Autodesk Inventor part; units mm, degrees
ref_plane "YZ Plane" through (0, 0, 0) normal (1, 0, 0) x (0, 1, 0)
ref_plane "XZ Plane" through (0, 0, 0) normal (0, 1, 0) x (-1, 0, 0)
sketch "Sketch1" plane through (0, 0, 0) normal (0, 1, 0) x (-1, 0, 0)
  line L0 (25.4, 127) -> (-25.4, 127)
  line L1 (-25.4, 127) -> (-25.4, -127)
  line L2 (-25.4, -127) -> (25.4, -127)
  line L3 (25.4, -127) -> (25.4, 127)
  line L4 (25.4, 127) -> (-25.4, -127) construction
  line L5 (-25.4, 127) -> (25.4, -127) construction
  point P0 (0, 0)
  dimension "d0" = 50.8
  dimension "d1" = 254
extrude "Extrusion1" add sketch "Sketch1" along normal blind 25.4
sketch "Sketch2" plane through (0, 0, 0) normal (0, -1, 0) x (1, 0, 0)
  line L0 (-25.4, 127) -> (-25.4, 114.3)
  line L1 (-25.4, 114.3) -> (25.4, 114.3)
  line L2 (25.4, 114.3) -> (25.4, 127)
  line L3 (25.4, 127) -> (-25.4, 127)
  line L4 (-25.4, 127) -> (25.4, 114.3) construction
  line L5 (-25.4, 114.3) -> (25.4, 127) construction
  line L6 (-25.4, 127) -> (25.4, 127)
  point P0 (0, 0)
  point P1 (0, 120.65)
  dimension "d4" = 12.7
  dimension "d5" = 25.4
  dimension "d6" = 0
extrude "Extrusion2" add sketch "Sketch2" along normal blind 6.35
mirror "Mirror1" about plane through (0, 0, 0) normal (0, 0, 1) of "Extrusion2"
sketch "Sketch3" plane through (0, 25.4, 0) normal (0, 1, 0) x (1, 0, 0)
  circle A0 centre (0, -88.9) radius 4.7625
  line L0 (-25.4, -127) -> (25.4, -127)
  point P0 (0, 0)
  dimension "d9" = 9.525
  dimension "d10" = 38.1
extrude "Extrusion3" cut sketch "Sketch3" against normal through all
mirror "Mirror2" about plane through (0, 0, 0) normal (0, 0, 1) of "Extrusion3"
sketch "Sketch4" plane through (0, 25.4, 0) normal (0, 1, 0) x (1, 0, 0)
  line L0 (-15.875, -76.2) -> (15.875, -76.2)
  line L1 (15.875, -76.2) -> (15.875, 76.2)
  line L2 (15.875, 76.2) -> (-15.875, 76.2)
  line L3 (-15.875, 76.2) -> (-15.875, -76.2)
  line L4 (-15.875, -76.2) -> (15.875, 76.2) construction
  line L5 (15.875, -76.2) -> (-15.875, 76.2) construction
  line L6 (-25.4, 127) -> (-25.4, -127)
  line L7 (-25.4, -127) -> (25.4, -127)
  point P0 (0, 0)
  dimension "d13" = 9.525
  dimension "d14" = 50.8
extrude "Extrusion4" cut sketch "Sketch4" against normal through all
properties part number "BandSawJigTop" material "LCP Plastic"
The model under review builds one solid part; all positions refer to its coordinate system, in mm. A direction names the side the tool comes from. Round coordinates to 2 decimals unless told otherwise and drop trailing zeros. Write each loop counter-clockwise with the first axis right and the second up, starting at its lowest first coordinate (ties: lowest second). Pieces come first, ordered by that corner, then holes. Notation, with made-up numbers: (56.5, -2.5) - (105.5, -2.5) arc R25 ccw to (105.5, 15.5) - close; hole circle Ø6 at (-32, 79.5). An arc over 180 degrees is marked (long way). One line per item, written item: value. Start each with the question number.
1. The part is to be moulded in two halves that separate along X. For faces 1 (the face through (0, 13, 76.2)), 2 (the face through (0, -3, 114.3)), 3 (the face through (15.875, 13, 1)), 4 (the face through (-25.4, 13, 2)), say which applies: released by +X, released by -X, zero draft, split by the parting line, or undercut.
2. Machinability: for faces 5 (the face through (-17, 25.4, 2)), 6 (the face through (0, 13, -76.2)), 7 (the face through (0, -3, -114.3)), which of the approach directions +Z, -Z, +X, -X, +Y, -Y give a long, thin tool a straight path to every point of the face, cutting with its end or side? Answer none if there is none.
3. Clearance check with a flat-ended pin moving along its axis: P1, Ø15, axis at x = 10.5, z = 26.5, coming from the -Y side. State where the tip first meets the part, or that it passes through.
4. Consider section D-D on y = -3. Write out the cut boundary in (x, z), and give its area (3 significant figures).
5. To check wall thickness, follow L1, parallel to Z at x = 0, y = 17.5; L2, parallel to X at y = 13, z = 35.5 (3 decimals); L3, parallel to Z at x = 11.5, y = -3. State the ranges of each line that lie inside material, in increasing order. Write a range as from..to.
6. Consider section C-C on y = 21. Write out the cut boundary in (x, z) (1 decimal).
7. Consider section B-B on z = -25. Write out the cut boundary in (x, y) (3 decimals).
8. Consider section A-A on x = 8. Write out the cut boundary in (y, z).
Checks:
1. face 1: undercut
1. face 2: zero draft
1. face 3: undercut
1. face 4: released by -X
2. face 5: +Z, -Z, +X, -X, +Y
2. face 6: +Y, -Y
2. face 7: +X, -X, -Y
3. P1: stops at y = 0
4. outline: (-25.4, -127) - (25.4, -127) - (25.4, -114.3) - (-25.4, -114.3) - close; (-25.4, 114.3) - (25.4, 114.3) - (25.4, 127) - (-25.4, 127) - close
4. area: 1,290 mm^2
5. L1: z = -127..-93.66, -84.14..-76.2, 76.2..84.14, 93.66..127
5. L2: x = -25.4..-15.875, 15.875..25.4
5. L3: z = -127..-114.3, 114.3..127
6. outline: (-25.4, -127) - (25.4, -127) - (25.4, 127) - (-25.4, 127) - close; hole (-15.9, -76.2) - (15.9, -76.2) - (15.9, 76.2) - (-15.9, 76.2) - close; hole circle Ø9.5 at (0, -88.9); hole circle Ø9.5 at (0, 88.9)
7. outline: (-25.4, 0) - (-15.875, 0) - (-15.875, 25.4) - (-25.4, 25.4) - close; (15.875, 0) - (25.4, 0) - (25.4, 25.4) - (15.875, 25.4) - close
8. outline: (-6.35, -127) - (25.4, -127) - (25.4, -76.2) - (0, -76.2) - (0, -114.3) - (-6.35, -114.3) - close; (-6.35, 114.3) - (0, 114.3) - (0, 76.2) - (25.4, 76.2) - (25.4, 127) - (-6.35, 127) - close
